```python
from build123d import *

# Parameters (mm, degrees)
PAD001_DEPTH            = 15
PAD_DEPTH               = 16
PAD002_DEPTH            = 3
PAD003_DEPTH            = 15
PAD001_MIRRORED_2_DEPTH = 15
PAD_MIRRORED_2_DEPTH    = 16
PAD002_MIRRORED_2_DEPTH = 3
PAD003_MIRRORED_2_DEPTH = 15
FILLET_R                = 3


with BuildPart() as part:
    # Sketch001 → Pad001 (new body)
    with BuildSketch(Plane(origin=(-41.5, 0, 0), x_dir=(-1, 0, 0), z_dir=(0, 1, 0))):
        Polygon((0, 0), (-1.5, -1.5), (0, -1.5), align=None)
    pad001 = extrude(amount=PAD001_DEPTH)

    # Sketch → Pad (join)
    with BuildSketch(Plane.XY):
        with BuildLine():
            Line((0, 36.5), (-37.5, 36.5))
            ThreePointArc((-37.5, 36.5), (-40.328427, 35.328427), (-41.5, 32.5))
            Line((-41.5, 32.5), (-41.5, 0))
            Line((-41.5, 0), (-44.5, 0))
            Line((-44.5, 0), (-44.5, 32.5))
            ThreePointArc((-37.5, 39.5), (-42.449747, 37.449747), (-44.5, 32.5))
            Line((-37.5, 39.5), (0, 39.5))
            Line((0, 36.5), (0, 39.5))
        make_face()
    pad = extrude(amount=-PAD_DEPTH)

    # Sketch002 (on Face14 of Pad) → Pad002 (join)
    with BuildSketch(Plane(origin=(-41.5, 0, -16), x_dir=(-1, 0, 0), z_dir=(0, 0, -1))):
        with BuildLine():
            Line((-41.5, 39.5), (-4, 39.5))
            ThreePointArc((3, 32.5), (0.949747, 37.449747), (-4, 39.5))
            Line((3, 32.5), (3, 0))
            Line((3, 0), (-41.5, 0))
            Line((-41.5, 0), (-41.5, 39.5))
        make_face()
    pad002 = extrude(amount=-PAD002_DEPTH)

    # Sketch003 (on Face6 of Pad002) → Pad003 (join)
    with BuildSketch(Plane(origin=(0, 36.5, 0), x_dir=(0, 1, 0), z_dir=(-1, 0, 0))):
        Polygon((0, 0), (-1.5, 1.5), (0, 1.5), align=None)
    pad003 = extrude(amount=PAD003_DEPTH)

    # Sketch001 Mirrored 2 → Pad001 Mirrored 2 (add)
    with BuildSketch(Plane(origin=(-41.5, 0, 0), x_dir=(-1, 0, 0), z_dir=(0, 1, 0))):
        Polygon((0, 0), (-1.5, -1.5), (0, -1.5), align=None)
    pad001_mirrored_2 = extrude(amount=-PAD001_MIRRORED_2_DEPTH)

    # Sketch Mirrored 2 → Pad Mirrored 2 (add)
    with BuildSketch(Plane(origin=(0, 0, 0), x_dir=(1, 0, 0), z_dir=(0, 0, -1))):
        with BuildLine():
            Line((0, 36.5), (-37.5, 36.5))
            ThreePointArc((-37.5, 36.5), (-40.328427, 35.328427), (-41.5, 32.5))
            Line((-41.5, 32.5), (-41.5, 0))
            Line((-41.5, 0), (-44.5, 0))
            Line((-44.5, 0), (-44.5, 32.5))
            ThreePointArc((-37.5, 39.5), (-42.449747, 37.449747), (-44.5, 32.5))
            Line((-37.5, 39.5), (0, 39.5))
            Line((0, 36.5), (0, 39.5))
        make_face()
    pad_mirrored_2 = extrude(amount=PAD_MIRRORED_2_DEPTH)

    # Sketch002 Mirrored 2 → Pad002 Mirrored 2 (add)
    with BuildSketch(Plane(origin=(-41.5, 0, -16), x_dir=(-1, 0, 0), z_dir=(0, 0, 1))):
        with BuildLine():
            Line((-41.5, 39.5), (-4, 39.5))
            ThreePointArc((3, 32.5), (0.949747, 37.449747), (-4, 39.5))
            Line((3, 32.5), (3, 0))
            Line((3, 0), (-41.5, 0))
            Line((-41.5, 0), (-41.5, 39.5))
        make_face()
    pad002_mirrored_2 = extrude(amount=PAD002_MIRRORED_2_DEPTH)

    # Sketch003 Mirrored 2 → Pad003 Mirrored 2 (add)
    with BuildSketch(Plane(origin=(0, -36.5, 0), x_dir=(0, -1, 0), z_dir=(1, 0, 0))):
        Polygon((0, 0), (-1.5, 1.5), (0, 1.5), align=None)
    pad003_mirrored_2 = extrude(amount=-PAD003_MIRRORED_2_DEPTH)

    # Mirrored001: Pad001, Pad, Pad002, Pad003, Pad001 Mirrored 2, Pad Mirrored 2, Pad002 Mirrored 2, Pad003 Mirrored 2 across YZ
    add(pad001.mirror(Plane.YZ))
    add(pad.mirror(Plane.YZ))
    add(pad002.mirror(Plane.YZ))
    add(pad003.mirror(Plane.YZ))
    add(pad001_mirrored_2.mirror(Plane.YZ))
    add(pad_mirrored_2.mirror(Plane.YZ))
    add(pad002_mirrored_2.mirror(Plane.YZ))
    add(pad003_mirrored_2.mirror(Plane.YZ))

    # Fillet
    fillet_edges = [part.edges().sort_by_distance(p)[0] for p in [
        (-41.5, 16.25, -13),
        (-40.328427, 35.328427, -13),
        (-18.75, 36.5, -13),
        (0, 18.25, -13),
        (-20.75, 0, -13),
        (41.5, 16.25, -13),
        (40.328427, 35.328427, -13),
        (18.75, 36.5, -13),
        (20.75, 0, -13),
        (41.5, -16.25, -13),
        (40.328427, -35.328427, -13),
        (18.75, -36.5, -13),
        (0, -18.25, -13),
        (-41.5, -16.25, -13),
        (-40.328427, -35.328427, -13),
        (-18.75, -36.5, -13),
    ]]
    fillet(fillet_edges, radius=FILLET_R)


solid = part.part
```
Input: part model. Units: mm. Frame: model coordinates. A direction names the side the tool comes from. Give positions to 0.01 mm unless a question says otherwise; leave off trailing zeros. Write each loop counter-clockwise with the first axis right and the second up, starting at its lowest first coordinate (ties: lowest second). Pieces come first, ordered by that corner, then holes. Notation, with made-up numbers: (20.25, 51) - (67.25, 51) arc R16 cw to (67.25, 55) - close; hole circle Ø2 at (51.25, 47). An arc over 180 degrees is marked (long way). Write item = value, one per line. Start each with the question number.
1. Section query A-A, the plane x = 35.5. Output: boundary loops of the cut face in (y, z).
2. Mould query, pull axis Z, two halves, no side actions, for faces 4 (the flat face through (-1, -1, -16)), 5 (the flat face through (-1, 36.5, -5)), 6 (the flat face through (0, -38, 0)), 7 (the cylindrical face through (42.4, 37.5, -7.9)). Classes: released by +Z, released by -Z, zero draft, split by the parting line, or undercut.
3. Section query D-D, the plane y = 24. Output: boundary loops of the cut face in (x, z).
4. Access query for faces 1 (the flat face through (44.5, 0, -8)), 2 (the cylindrical face through (-40.297, 35.359, -4.93)), 3 (the flat face through (-41.5, 0, -5)). Directions: +Z, -Z, +X, -X, +Y, -Y. A direction counts if a zero-diameter tool reaches every point of the face in a straight line with its end or side. Return the directions, or none.
5. Section query C-C, the plane y = -7. Output: boundary loops of the cut face in (x, z).
6. Section query B-B, the plane z = -4. Output: boundary loops of the cut face in (x, y), then the cut area to 3 significant figures.
7. Ray query, L1, parallel to X at y = 12.5, z = -4; L2, parallel to Y at x = -17, z = -3.25; L3, parallel to Z at x = 8, y = 4. Return the intervals inside material, ascending.
8. First-contact query: pin 1 Ø1.2 at (y, z) = (-35.5, -1) entering from -X; pin 2 Ø0.8 at (x, z) = (-40.5, -1) entering from -Y; pin 3 Ø1.6 at (y, z) = (-35.5, -0.5) entering from +X. Flat tips, straight axial feed; report the tip coordinate or a pass-through.
Check sheet entries:
q1.outline = (-39.5, -16) - (39.5, -16) - (39.5, 0) - (36.5, 0) - (36.5, -10) arc R3 cw to (33.5, -13) - (-33.5, -13) arc R3 cw to (-36.5, -10) - (-36.5, 0) - (-39.5, 0) - close
q2.face_4 = released by -Z
q2.face_5 = undercut
q2.face_6 = released by +Z
q2.face_7 = zero draft
q3.outline = (-44.5, -16) - (44.5, -16) - (44.5, 0) - (41.5, 0) - (41.5, -10) arc R3 cw to (38.5, -13) - (-38.5, -13) arc R3 cw to (-41.5, -10) - (-41.5, 0) - (-44.5, 0) - close
q4.face_1 = +Z, -Z, +X, +Y, -Y
q4.face_2 = +Z
q4.face_3 = none
q5.outline = (-44.5, -16) - (44.5, -16) - (44.5, 0) - (41.5, 0) - (40, -1.5) - (41.5, -1.5) - (41.5, -10) arc R3 cw to (38.5, -13) - (-38.5, -13) arc R3 cw to (-41.5, -10) - (-41.5, -1.5) - (-40, -1.5) - (-41.5, 0) - (-44.5, 0) - close
q6.outline = (-44.5, -32.5) arc R7 ccw to (-37.5, -39.5) - (37.5, -39.5) arc R7 ccw to (44.5, -32.5) - (44.5, 32.5) arc R7 ccw to (37.5, 39.5) - (-37.5, 39.5) arc R7 ccw to (-44.5, 32.5) - close; hole (-41.5, -32.5) arc R4 ccw to (-37.5, -36.5) - (37.5, -36.5) arc R4 ccw to (41.5, -32.5) - (41.5, 32.5) arc R4 ccw to (37.5, 36.5) - (-37.5, 36.5) arc R4 ccw to (-41.5, 32.5) - close
q6.area = 944 mm2
q7.L1 = -44.5 to -41.5, 41.5 to 44.5
q7.L2 = -39.5 to -36.5, 36.5 to 39.5
q7.L3 = -16 to -13
q8.pin_1 = -44.08
q8.pin_2 = -39
q8.pin_3 = 44.15
